Read the model definition and answer for the solid it produces. Units are mm, in the model's axes. A direction names the side the tool comes from. Coordinates: 2 decimals unless noted, no trailing zeros. Order: outer loops, then holes, each group sorted by start corner. A loop starts at its lowest first (then second) coordinate and runs counter-clockwise, first axis right, second up. Notation, with made-up numbers: M 63,68 L 69,68 A36 ccw 69,105 Z; hole C 18.25,80 d3. An arc over 180 degrees is marked long. Write each question's results on one line, items separated by ' | '.
Autodesk Inventor part; units mm, degrees
ref_plane "YZ Plane" through (0, 0, 0) normal (1, 0, 0) x (0, 1, 0)
ref_plane "XZ Plane" through (0, 0, 0) normal (0, 1, 0) x (-1, 0, 0)
ref_plane "XY Plane" through (0, 0, 0) normal (0, 0, 1) x (1, 0, 0)
sketch "Sketch1" plane through (0, 0, 0) normal (0, 1, 0) x (-1, 0, 0)
  line L0 (0, 0) -> (-76.2, 0)
  line L1 (-76.2, 0) -> (-76.2, -50.8)
  line L2 (-76.2, -50.8) -> (0, -50.8)
  line L3 (0, -50.8) -> (0, 0)
  dimension "d0" = 76.2
  dimension "d1" = 50.8
extrude "Extrusion1" add sketch "Sketch1" along normal blind 12.7
sketch "Sketch5" plane through (76.2, 0, -50.8) normal (0, 0, -1) x (-1, 0, 0)
  line L0 (76.2, 0) -> (73.66, 0)
  line L1 (76.2, 0) -> (0, 0)
  line L2 (73.66, 0) -> (53.34, 0)
  line L3 (53.34, 0) -> (58.42, 8.7988)
  line L4 (58.42, 8.7988) -> (68.58, 8.7988)
  line L5 (68.58, 8.7988) -> (73.66, 0)
  dimension "d9" = 2.54
  dimension "d10" = 20.32
  dimension "d11" = 10.16
  dimension "d12" = 60
  dimension "d13" = 10.16
extrude "Extrusion2" add sketch "Sketch5" along normal blind 2.54
sketch "Sketch6" plane through (76.2, 12.7, -50.8) normal (0, 0, -1) x (-1, 0, 0)
  line L0 (76.2, -12.7) -> (0, -12.7)
  line L1 (0, -12.7) -> (2.54, -12.7)
  line L2 (2.54, -12.7) -> (22.86, -12.7)
  line L3 (22.86, -12.7) -> (17.78, -3.9012)
  line L4 (17.78, -3.9012) -> (7.62, -3.9012)
  line L5 (7.62, -3.9012) -> (2.54, -12.7)
  dimension "d16" = 2.54
  dimension "d17" = 20.32
  dimension "d18" = 10.16
  dimension "d19" = 60
  dimension "d20" = 10.16
extrude "Extrusion3" add sketch "Sketch6" along normal blind 2.54
sketch "Sketch7" plane through (0, 0, 0) normal (0, 0, 1) x (1, 0, 0)
  line L0 (2.54, 0) -> (0, 0)
  line L1 (0, 0) -> (2.54, 0)
  line L2 (22.86, 0) -> (2.54, 0)
  line L3 (2.54, 0) -> (22.86, 0)
  line L4 (22.86, 0) -> (17.78, 8.7988)
  line L5 (22.86, 0) -> (17.78, 8.7988)
  line L6 (17.78, 8.7988) -> (7.62, 8.7988)
  line L7 (17.78, 8.7988) -> (7.62, 8.7988)
  line L8 (7.62, 8.7988) -> (2.54, 0)
  line L9 (7.62, 8.7988) -> (2.54, 0)
  dimension "d23" = 20.32
  dimension "d24" = 10.16
  dimension "d25" = 60
extrude "Extrusion4" add sketch "Sketch7" along normal blind 2.54
sketch "Sketch8" plane through (0, 12.7, 0) normal (0, 0, 1) x (1, 0, 0)
  line L0 (76.2, -12.7) -> (73.66, -12.7)
  line L1 (76.2, -12.7) -> (73.66, -12.7)
  line L2 (53.34, -12.7) -> (58.42, -3.9012)
  line L3 (73.66, -12.7) -> (53.34, -12.7)
  line L4 (53.34, -12.7) -> (58.42, -3.9012)
  line L5 (58.42, -3.9012) -> (68.58, -3.9012)
  line L6 (68.58, -3.9012) -> (73.66, -12.7)
  line L7 (68.58, -3.9012) -> (73.66, -12.7)
  point P0 (0, -12.7)
  dimension "d28" = 10.16
extrude "Extrusion5" add sketch "Sketch8" along normal blind 2.54
sketch "Sketch10" plane through (76.2, 12.7, -53.34) normal (0, 0, -1) x (-1, 0, 0)
  line L0 (7.62, -3.9012) -> (2.54, -12.7)
  line L1 (2.54, -12.7) -> (12.7, -12.7)
  line L2 (2.54, -12.7) -> (22.86, -12.7)
  line L3 (2.54, -12.7) -> (4.318, -12.7)
  line L4 (4.318, -12.7) -> (8.509, -5.441)
  line L5 (8.509, -5.441) -> (16.891, -5.441)
  line L6 (16.891, -5.441) -> (21.082, -12.7)
  line L7 (21.082, -12.7) -> (16.891, -19.959)
  line L8 (16.891, -19.959) -> (8.509, -19.959)
  line L9 (8.509, -19.959) -> (4.318, -12.7)
  point P0 (76.2, -12.7)
  dimension "d31" = 1.778
extrude "Extrusion6" cut sketch "Sketch10" against normal blind 7.62
sketch "Sketch11" plane through (76.2, 0, -53.34) normal (0, 0, -1) x (-1, 0, 0)
  line L0 (53.34, 0) -> (73.66, 0)
  line L1 (53.34, 0) -> (63.5, 0)
  line L2 (22.86, 0) -> (53.34, 0)
  line L3 (53.34, 0) -> (55.118, 0)
  line L4 (55.118, 0) -> (59.309, 7.259)
  line L5 (59.309, 7.259) -> (67.691, 7.259)
  line L6 (67.691, 7.259) -> (71.882, 0)
  line L7 (71.882, 0) -> (67.691, -7.259)
  line L8 (67.691, -7.259) -> (59.309, -7.259)
  line L9 (59.309, -7.259) -> (55.118, 0)
  point P0 (76.2, 0)
  dimension "d34" = 10.16
  dimension "d35" = 1.778
extrude "Extrusion7" cut sketch "Sketch11" against normal blind 7.62
sketch "Sketch12" plane through (0, 0, 2.54) normal (0, 0, 1) x (1, 0, 0)
  line L0 (0, 0) -> (2.54, 0)
  line L1 (2.54, 0) -> (12.7, 0)
  line L2 (2.54, 0) -> (22.86, 0)
  line L3 (2.54, 0) -> (4.318, 0)
  line L4 (4.318, 0) -> (8.509, 7.259)
  line L5 (8.509, 7.259) -> (16.891, 7.259)
  line L6 (16.891, 7.259) -> (21.082, 0)
  line L7 (21.082, 0) -> (16.891, -7.259)
  line L8 (16.891, -7.259) -> (8.509, -7.259)
  line L9 (8.509, -7.259) -> (4.318, 0)
  dimension "d38" = 10.16
  dimension "d39" = 1.778
extrude "Extrusion8" cut sketch "Sketch12" against normal blind 7.62
sketch "Sketch13" plane through (0, 12.7, 2.54) normal (0, 0, 1) x (1, 0, 0)
  line L0 (22.86, -12.7) -> (53.34, -12.7)
  line L1 (53.34, -12.7) -> (63.5, -12.7)
  line L2 (53.34, -12.7) -> (73.66, -12.7)
  line L3 (53.34, -12.7) -> (55.118, -12.7)
  line L4 (55.118, -12.7) -> (59.309, -5.441)
  line L5 (59.309, -5.441) -> (67.691, -5.441)
  line L6 (67.691, -5.441) -> (71.882, -12.7)
  line L7 (71.882, -12.7) -> (67.691, -19.959)
  line L8 (67.691, -19.959) -> (59.309, -19.959)
  line L9 (59.309, -19.959) -> (55.118, -12.7)
  point P0 (0, -12.7)
  dimension "d42" = 10.16
  dimension "d43" = 1.778
extrude "Extrusion9" cut sketch "Sketch13" against normal blind 7.62
properties part number "tesla v2"
(1) The part is cut by section C-C, the plane x = 56. Write down the section's boundary in (y, z).
Conclusion:
outline: M 0,-45.72 L 1.53,-45.72 L 1.53,-53.34 L 4.61,-53.34 L 4.61,-50.8 L 12.7,-50.8 L 12.7,0 L 4.61,0 L 4.61,2.54 L 1.53,2.54 L 1.53,-5.08 L 0,-5.08 Z
(2) Straight lines are drawn through the part: line 1 (Z direction, x = 52, y = 5.5); line 2 (Z direction, x = 59, y = 1); line 3 (Y direction, x = 69, z = -48.5). For each, find the intervals that lie inside material, in ascending order.
Conclusion:
line 1: -50.8 to 0 | line 2: -45.72 to -5.08 | line 3: 4.99 to 12.7
(3) The mould has two halves that part along X. Classify faces 6 (the flat face through (39, 8, -50.8)), 7 (the flat face through (14, 8, -53.34)), 8 (the flat face through (71.084, 4.461, 1.252)): pulls with the +X half, pulls with the -X half, needs draft (parallel to the pull), parting line crosses it, or undercut.
Conclusion:
face 6: undercut | face 7: needs draft | face 8: pulls with the +X half
(4) Given pin 1 (2 mm diameter, centred on x = 64.5, y = 3.5, fed in from -Z); pin 2 (4 mm diameter, centred on x = 64.5, z = -50, fed in from -Y); pin 3 (2 mm diameter, centred on x = 62.5, z = -52.5, fed in from +Y); pin 4 (1.5 mm diameter, centred on y = 11.5, z = -47, fed in from -X), each flat-ended and moving along its own axis, determine where each tip first touches the part or whether it passes through.
Conclusion:
pin 1: z = -45.72 | pin 2: y = 7.26 | pin 3: y = 8.8 | pin 4: x = 0
(5) The part is cut by section A-A, the plane x = 14.5. Write down the section's boundary in (y, z).
Conclusion:
outline: M 0,-45.72 L 7.26,-45.72 L 7.26,-53.34 L 8.8,-53.34 L 8.8,-50.8 L 12.7,-50.8 L 12.7,0 L 8.8,0 L 8.8,2.54 L 7.26,2.54 L 7.26,-5.08 L 0,-5.08 Z
(6) The part is cut by section D-D, the plane x = 37. Write down the section's boundary in (y, z), then the cut area to 3 significant figures.
Conclusion:
outline: M 0,-50.8 L 12.7,-50.8 L 12.7,0 L 0,0 Z | area: 645 mm²
(7) The part is cut by section B-B, the plane y = 11.5. Write down the section's boundary in (x, z).
Conclusion:
outline: M 0,-50.8 L 76.2,-50.8 L 76.2,0 L 0,0 Z
(8) For faces 1 (the flat face through (63, 8.799, -52)), 2 (the flat face through (69.816, 3.579, -49.583)), 3 (the flat face through (71.084, 4.461, -52.052)), 4 (the flat face through (69.757, 3.68, -1.217)), 5 (the flat face through (55.844, 4.338, -52.052)), determine the directions among +Z, -Z, +X, -X, +Y, -Y from which every point of the face is accessible in a straight line to the end or side of a thin tool.
Conclusion:
face 1: -Z, +X, -X, +Y | face 2: -Z, -Y | face 3: -Z, +X, +Y | face 4: +Z, -Y | face 5: -Z, +Y
